Verification items for the finished model (mm, model axes). A direction names the side the tool comes from. Coordinates: 2 decimals unless noted, no trailing zeros. Order: outer loops, then holes, each group sorted by start corner. A loop starts at its lowest first (then second) coordinate and runs counter-clockwise, first axis right, second up. Notation, with made-up numbers: (-23.75, 26.25) -> (23.25, 26.25) arc R28 cw to (23.25, 54.25) -> close; hole circle Ø10 at (-25.75, 38.25). An arc over 180 degrees is marked (long way). Write item = value, one per line. Start each with the question number.
1. Set-up check for faces 1 (the flat face through (5.08, -3, 46)), 2 (the flat face through (3, -3, 45.085)), 3 (the flat face through (96.8, 0.2, 29.2)): record each of +Z, -Z, +X, -X, +Y, -Y from which the full face is reachable in a straight line by a thin tool's end or side.
2. Cross-section at A-A on y = -3.5. Record the cut outline in (x, z) (3 decimals), plus the area to 3 significant figures.
3. Cross-section at C-C on z = 32. Record the cut outline in (x, y), plus the area to 3 significant figures.
4. Thickness scan on line 1 along Y through (x, z) = (31, 29); line 2 along Z through (x, y) = (93.5, -0.75) (3 decimals). Record the ranges inside material, lowest first. Write a range as from..to.
5. Release check for a two-part mould opening along Z. For faces 4 (the flat face through (48.6, 0.4, 47.625)), 5 (the flat face through (94, -3, 45.085)), 6 (the cylindrical face through (40.806, 0.618, 42.445)) record: +Z half, -Z half, draft (parallel to the pull), parting line (faces both ways), or undercut.
6. Go/stop test with flat-tipped pins: P1, Ø3, axis at x = 65, z = 13, coming from the -Y side; P2, Ø1.4, axis at x = 40.46, z = 7.54, coming from the -Y side; P3, Ø1.5, axis at x = 28, y = -0.5, coming from the -Z side. Record where each tip stops, or that it passes through.
7. Cross-section at B-B on x = 16.5. Record the cut outline in (y, z) (3 decimals).
from build123d import *

# Parameters (mm, degrees)
SKETCH1_W           = 96.799999948
SKETCH1_H           = 47.62500254
BOSS_EXTRUDE1_DEPTH = 1.2192
CUT_EXTRUDE1_REACH  = 109.888
SKETCH5_R           = 1.143
CUT_EXTRUDE2_REACH  = 109.888
SKETCH6_R           = 1.143
SKETCH7_W           = 5.08
SKETCH7_H           = 2.54
BOSS_EXTRUDE2_DEPTH = 5.08


with BuildPart() as part:
    # Sketch1 → Boss-Extrude1 (new body)
    with BuildSketch(Plane(origin=(0, 0, 0), x_dir=(1, 0, 0), z_dir=(0, 1, 0))):
        with Locations((48.399999974, -23.81250127)):
            Rectangle(SKETCH1_W, SKETCH1_H)
    extrude(amount=BOSS_EXTRUDE1_DEPTH)

    # Sketch5 → Cut-Extrude1 (cut, up to next)
    with BuildSketch(Plane(origin=(0, 1.2192, 0), x_dir=(1, 0, 0), z_dir=(0, 1, 0)), mode=Mode.PRIVATE) as cut_extrude1_sk1:
        with Locations(Location((56.3375, -7.540625, 0), (0, 0, 270))):
            Circle(SKETCH5_R)
    cut_extrude1_tool1 = extrude(cut_extrude1_sk1.sketch, amount=-CUT_EXTRUDE1_REACH, mode=Mode.PRIVATE) & part.part
    # Sketch5 → Cut-Extrude1 (cut, up to next)
    with BuildSketch(Plane(origin=(0, 1.2192, 0), x_dir=(1, 0, 0), z_dir=(0, 1, 0)), mode=Mode.PRIVATE) as cut_extrude1_sk2:
        with Locations(Location((40.4625, -7.540625, 0), (0, 0, 270))):
            Circle(SKETCH5_R)
    cut_extrude1_tool2 = extrude(cut_extrude1_sk2.sketch, amount=-CUT_EXTRUDE1_REACH, mode=Mode.PRIVATE) & part.part
    add(cut_extrude1_tool1.solids().sort_by_distance((56.3375, 1.2192, 7.540625))[0], mode=Mode.SUBTRACT)
    add(cut_extrude1_tool2.solids().sort_by_distance((40.4625, 1.2192, 7.540625))[0], mode=Mode.SUBTRACT)

    # Sketch6 → Cut-Extrude2 (cut, up to next)
    with BuildSketch(Plane(origin=(0, 1.2192, 0), x_dir=(1, 0, 0), z_dir=(0, 1, 0)), mode=Mode.PRIVATE) as cut_extrude2_sk1:
        with Locations(Location((56.3375, -41.35437754, 0), (0, 0, 270))):
            Circle(SKETCH6_R)
    cut_extrude2_tool1 = extrude(cut_extrude2_sk1.sketch, amount=-CUT_EXTRUDE2_REACH, mode=Mode.PRIVATE) & part.part
    # Sketch6 → Cut-Extrude2 (cut, up to next)
    with BuildSketch(Plane(origin=(0, 1.2192, 0), x_dir=(1, 0, 0), z_dir=(0, 1, 0)), mode=Mode.PRIVATE) as cut_extrude2_sk2:
        with Locations(Location((40.4625, -41.35437754, 0), (0, 0, 270))):
            Circle(SKETCH6_R)
    cut_extrude2_tool2 = extrude(cut_extrude2_sk2.sketch, amount=-CUT_EXTRUDE2_REACH, mode=Mode.PRIVATE) & part.part
    add(cut_extrude2_tool1.solids().sort_by_distance((56.3375, 1.2192, 41.354378))[0], mode=Mode.SUBTRACT)
    add(cut_extrude2_tool2.solids().sort_by_distance((40.4625, 1.2192, 41.354378))[0], mode=Mode.SUBTRACT)

    # Sketch7 → Boss-Extrude2 (add)
    with BuildSketch(Plane(origin=(0, 0, 0), x_dir=(-1, 0, 0), z_dir=(0, -1, 0))):
        with Locations((-94.259999948, -46.35500254)):
            Rectangle(SKETCH7_W, SKETCH7_H)
        with Locations((-2.54, -46.35500254)):
            Rectangle(SKETCH7_W, SKETCH7_H)
    extrude(amount=BOSS_EXTRUDE2_DEPTH)


solid = part.part
Worked out:
q1.face_1 = +Z, -Z, -Y
q1.face_2 = -Z, +X, -X, -Y
q1.face_3 = +Z, -Z, +X, +Y, -Y
q2.outline = (0, 45.085) -> (5.08, 45.085) -> (5.08, 47.625) -> (0, 47.625) -> close; (91.72, 45.085) -> (96.8, 45.085) -> (96.8, 47.625) -> (91.72, 47.625) -> close
q2.area = 25.8 mm²
q3.outline = (0, 0) -> (96.8, 0) -> (96.8, 1.22) -> (0, 1.22) -> close
q3.area = 118 mm²
q4.line_1 = 0..1.22
q4.line_2 = 45.085..47.625
q5.face_4 = +Z half
q5.face_5 = -Z half
q5.face_6 = undercut
q6.P1 = 0
q6.P2 = through
q6.P3 = 0
q7.outline = (0, 0) -> (1.219, 0) -> (1.219, 47.625) -> (0, 47.625) -> close
